Geometry: see drawing. Coordinates: mm, zero at the bounding-box minimum. Round coordinates to 2 decimals unless told otherwise and drop trailing zeros. Write each loop counter-clockwise with the first axis right and the second up, starting at its lowest first coordinate (ties: lowest second). Pieces come first, ordered by that corner, then holes.
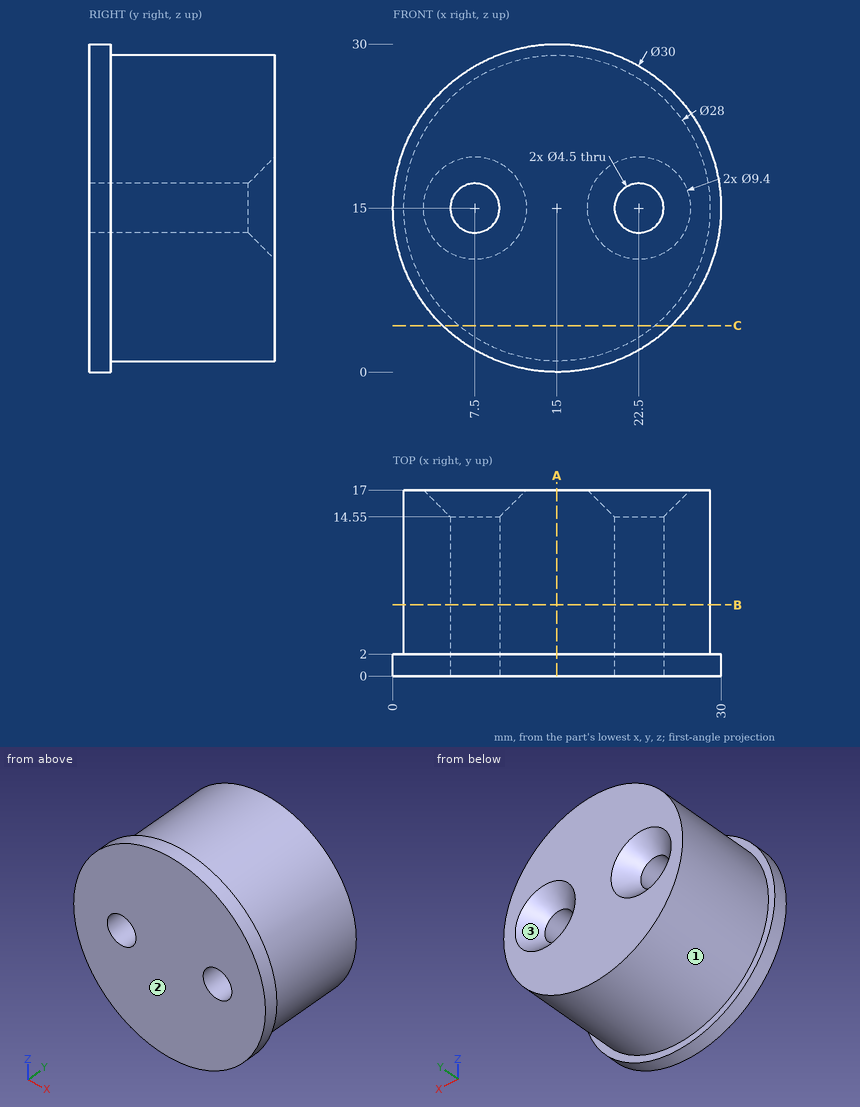
Q1. Section query C-C, the plane z = 4.25. Output: boundary loops of the cut face in (x, y).
Q2. Line query: line 1 (X direction, y = 1.5, z = 16.75); line 2 (Z direction, x = 22.5, y = 6.5); line 3 (X direction, y = 8.5, z = 14). Output: solid intervals per line, ascending.
Q3. Section query A-A, the plane x = 15. Output: boundary loops of the cut face in (y, z), and give its area (3 significant figures).
Q4. Section query B-B, the plane y = 6.5. Output: boundary loops of the cut face in (x, z).
Q5. Pin query (flat end, axial travel): P1, Ø3, axis at y = 14.5, z = 4, coming from the -X side; P2, Ø3, axis at x = 26.5, y = 12, coming from the -Z side; P3, Ø1, axis at x = 5.5, y = 7, coming from the -Z side. Return the tip coordinate at first contact, or that it passes through.
Q6. Mould query, pull axis Z, two halves, no side actions, for the marked faces 1, 2 and 3. Classes: pulls with the +Z half, pulls with the -Z half, needs draft (parallel to the pull), parting line crosses it, or undercut.
Filled in:
1. outline: (4.54, 0) - (25.46, 0) - (25.46, 2) - (23.97, 2) - (23.97, 17) - (6.03, 17) - (6.03, 2) - (4.54, 2) - close
2. line 1: x = 0.1 to 6.09, 8.91 to 21.09, 23.91 to 29.9
2. line 2: z = 3.18 to 12.75, 17.25 to 26.82
2. line 3: x = 1.04 to 5.48, 9.52 to 20.48, 24.52 to 28.96
3. outline: (0, 0) - (2, 0) - (2, 1) - (17, 1) - (17, 29) - (2, 29) - (2, 30) - (0, 30) - close
3. area: 480 mm2
4. outline: circle Ø28 at (15, 15); hole circle Ø4.5 at (7.5, 15); hole circle Ø4.5 at (22.5, 15)
5. P1: stops at x = 4.72
5. P2: stops at z = 5.2
5. P3: stops at z = 4.28
6. face 1: parting line crosses it
6. face 2: needs draft
6. face 3: undercut
